```python
from build123d import *

# Parameters (mm, degrees)
BOSS_EXTRUDE1_DEPTH = 10
BOSS_EXTRUDE2_DEPTH = 8
BOSS_EXTRUDE4_DEPTH = 25
SKETCH3_W           = 12.484022429
SKETCH3_H           = 6.213790253
CUT_EXTRUDE1_DEPTH  = 8
SKETCH7_R           = 2.934045285
CUT_EXTRUDE4_DEPTH  = 18
SKETCH8_R           = 2.590039353
CUT_EXTRUDE5_DEPTH  = 18


with BuildPart() as part:
    # Sketch1 → Boss-Extrude1 (new body)
    with BuildSketch(Plane(origin=(0, 0, 0), x_dir=(1, 0, 0), z_dir=(0, 1, 0))):
        Polygon((27.346217797, 0), (37.346217797, 10), (37.346217797, 43.13883642), (0, 43.13883642), (0, 0), align=None)
    extrude(amount=BOSS_EXTRUDE1_DEPTH)

    # 3DSketch1 → Boss-Extrude2 (add)
    with BuildSketch(Plane(origin=(0, 10, -32.014495021), x_dir=(0.4303839412255019, 0, 0.9026459234579215), z_dir=(0, 1, 0))):
        Polygon((0, 0), (6.569636602, 13.778524544), (35.467390024, 0), (28.897753422, -13.778524544), align=None)
    extrude(amount=BOSS_EXTRUDE2_DEPTH)

    # Sketch2 → Boss-Extrude4 (add)
    with BuildSketch(Plane(origin=(0, 0, 0), x_dir=(1, 0, 0), z_dir=(0, 1, 0))):
        Polygon((0, 43.13883642), (37.346217797, 43.13883642), (37.346217797, 36.988423425), (32.346217797, 31.988423425), (0, 31.988423425), align=None)
    extrude(amount=BOSS_EXTRUDE4_DEPTH)

    # Sketch3 → Cut-Extrude1 (cut)
    with BuildSketch(Plane(origin=(0, 18, 0), x_dir=(1, 0, 0), z_dir=(0, 1, 0))):
        with Locations((9.02258389, 3.106895126)):
            Rectangle(SKETCH3_W, SKETCH3_H)
    extrude(amount=-CUT_EXTRUDE1_DEPTH, mode=Mode.SUBTRACT)

    # Sketch7 → Cut-Extrude4 (cut)
    with BuildSketch(Plane(origin=(0, 18, 0), x_dir=(1, 0, 0), z_dir=(0, 1, 0))):
        with Locations(Location((7.23477268, 26.681503573, 0), (0, 0, 270))):
            Circle(SKETCH7_R)
    extrude(amount=-CUT_EXTRUDE4_DEPTH, mode=Mode.SUBTRACT)

    # Sketch8 → Cut-Extrude5 (cut)
    with BuildSketch(Plane.XY.offset(-31.988423425)):
        with Locations((23.773325806, 17.384751646)):
            Circle(SKETCH8_R)
    extrude(amount=-CUT_EXTRUDE5_DEPTH, mode=Mode.SUBTRACT)


solid = part.part
```
Design review of the part built by this model. Coordinates are the model's own, in mm. A direction names the side the tool comes from. Give positions to 0.01 mm unless a question says otherwise; leave off trailing zeros. Write each loop counter-clockwise with the first axis right and the second up, starting at its lowest first coordinate (ties: lowest second). Pieces come first, ordered by that corner, then holes. Notation, with made-up numbers: (51.5, -2) - (82.5, -2) arc R21 ccw to (82.5, 16) - close; hole circle Ø1 at (29, 84.5). An arc over 180 degrees is marked (long way). Return JSON: item names as keys, results as strings. Group by question number.
(1) We need section D-D, the plane x = 17.5. Give the boundary of the cut face in (y, z), then the cut area to 3 significant figures.
(2) We need section C-C, the plane z = -35.5. Give the boundary of the cut face in (x, y).
(3) Machinability: for faces 4 (the flat face through (9, 14, -6.214)), 5 (the flat face through (19, 12, -43.139)), which of the approach directions +Z, -Z, +X, -X, +Y, -Y give a long, thin tool a straight path to every point of the face, cutting with its end or side? Answer none if there is none.
(4) We need section A-A, the plane x = 8. Give the boundary of the cut face in (y, z), then the cut area to 3 significant figures.
(5) Insertion check: pin 1 (4 mm diameter, centred on x = 8, y = 13, fed in from +Z); pin 2 (17.5 mm diameter, centred on x = 18, z = -16.5, fed in from +Y); pin 3 (3 mm diameter, centred on y = 14, z = -2, fed in from +X); pin 4 (4.5 mm diameter, centred on x = 7.23, z = -26.68, fed in from +Y). Each pin has a flat end and moves straight along its axis. Give the tip position at first contact, or say it passes through.
(6) We need section B-B, the plane y = 18.5. Give the boundary of the cut face in (x, z), then the cut area to 3 significant figures.
(7) To check wall thickness, follow probe 1 along X at (y, z) = (4.5, -26.5); probe 2 along Y at (x, z) = (19, -24); probe 3 along Z at (x, y) = (24, 21.5). State the ranges of each line that lie inside material, in increasing order.
(8) Mouldability with a two-part tool opening along X and no side actions: class faces 1 (the cylindrical face through (25.166, 19.569, -37.486)), 2 (the flat face through (15.265, 14, -19)), 3 (the flat face through (7, 18, -18)) as +X half, -X half, draft (parallel to the pull), parting line (faces both ways), or undercut.
Reported:
{
 "1": {"outline": "(0, -43.14) - (25, -43.14) - (25, -31.99) - (10, -31.99) - (10, 0) - (0, 0) - close", "area": "599 mm2"},
 "2": {"outline": "(0, 0) - (37.35, 0) - (37.35, 10) - (35.86, 10) - (35.86, 25) - (0, 25) - close; hole circle Ø5.18 at (23.77, 17.38)"},
 "3": {"face 4": "+Z, +X, +Y", "face 5": "-Z, +X, -X, +Y, -Y"},
 "4": {"outline": "(0, -43.14) - (25, -43.14) - (25, -31.99) - (18, -31.99) - (18, -29.51) - (0, -29.51) - close; (0, -23.85) - (18, -23.85) - (18, -6.21) - (10, -6.21) - (10, 0) - (0, 0) - close", "area": "703 mm2"},
 "5": {"pin 1": "stops at z = -6.21", "pin 2": "stops at y = 18", "pin 3": "stops at x = 2.78", "pin 4": "passes through"},
 "6": {"outline": "(0, -43.14) - (21.44, -43.14) - (21.44, -31.99) - (0, -31.99) - close; (26.11, -43.14) - (37.35, -43.14) - (37.35, -36.99) - (32.35, -31.99) - (26.11, -31.99) - close", "area": "352 mm2"},
 "7": {"probe 1": "x = 0 to 4.31, 10.16 to 37.35", "probe 2": "y = 0 to 10", "probe 3": "z = -43.14 to -31.99"},
 "8": {"face 1": "undercut", "face 2": "+X half", "face 3": "draft"}
}
